Autodesk Inventor part; units mm, degrees
ref_plane "YZ Plane" through (0, 0, 0) normal (1, 0, 0) x (0, 1, 0)
ref_plane "XZ Plane" through (0, 0, 0) normal (0, 1, 0) x (-1, 0, 0)
ref_plane "XY Plane" through (0, 0, 0) normal (0, 0, 1) x (1, 0, 0)
sketch "Sketch1" plane through (0, 0, 0) normal (0, 1, 0) x (-1, 0, 0)
  line L0 (0, 0) -> (0, -88.9)
  line L1 (0, -88.9) -> (-101.6, -88.9)
  line L2 (-101.6, -88.9) -> (-101.6, 0)
  line L3 (-101.6, 0) -> (0, 0)
  dimension "d0" = 88.9
  dimension "d1" = 101.6
extrude "Extrusion1" add sketch "Sketch1" along normal blind 12.7
sketch "Sketch2" plane through (0, 12.7, 0) normal (0, 1, 0) x (1, 0, 0)
  line L0 (101.6, 88.9) -> (0, 88.9)
  line L1 (0, 0) -> (12.7, 0)
  line L2 (12.7, 0) -> (12.7, 88.9)
  line L3 (12.7, 88.9) -> (0, 88.9)
  line L4 (0, 88.9) -> (0, 0)
  dimension "d4" = 12.7
extrude "Extrusion2" add sketch "Sketch2" along normal blind 88.9
properties part number "Post Bracket"
Design review of the part built by this model. Coordinates are the model's own, in mm. A direction names the side the tool comes from. Coordinates: 2 decimals unless noted, no trailing zeros. Loops run counter-clockwise (first coordinate to the right, second up) from the corner with the lowest first, then second, coordinate; pieces in that order, holes last. Notation, with made-up numbers: M 6.25,-23.5 L 26.25,-23.5 A22 ccw 26.25,-11.5 Z; hole C 69,48.25 d3. An arc over 180 degrees is marked long. Answer as CSV lines item,"result".
Item 1: Add section B-B on y = 55. State the section outline as (x, z) points, plus the area to 3 significant figures.
Answer list:
outline,"M 0,-88.9 L 12.7,-88.9 L 12.7,0 L 0,0 Z"
area,"1,130 mm²"
Item 2: Machinability: for faces 1 (the face through (52, 0, -44)), 2 (the face through (12.7, 57, -44)), which of the approach directions +Z, -Z, +X, -X, +Y, -Y give a long, thin tool a straight path to every point of the face, cutting with its end or side? Answer none if there is none.
Answer list:
face 1,"+Z, -Z, +X, -X, -Y"
face 2,"+Z, -Z, +X, +Y"
Item 3: For probe 1 along X at (y, z) = (90, -64), list the stretches that pass through material, from the lowest coordinate up.
Answer list:
probe 1,"0 to 12.7"
Item 4: Add section A-A on z = -77.5. State the section outline as (x, y) points, plus the area to 3 significant figures.
Answer list:
outline,"M 0,0 L 101.6,0 L 101.6,12.7 L 12.7,12.7 L 12.7,101.6 L 0,101.6 Z"
area,"2,420 mm²"
Item 5: For P1, Ø2, axis at x = 41.5, z = -43.5, coming from the +Y side; P2, Ø4, axis at x = 13, z = -35, coming from the +Y side, all flat-tipped, find the tip position at first contact; note any pin that passes through.
Answer list:
P1,"y = 12.7"
P2,"y = 101.6"
